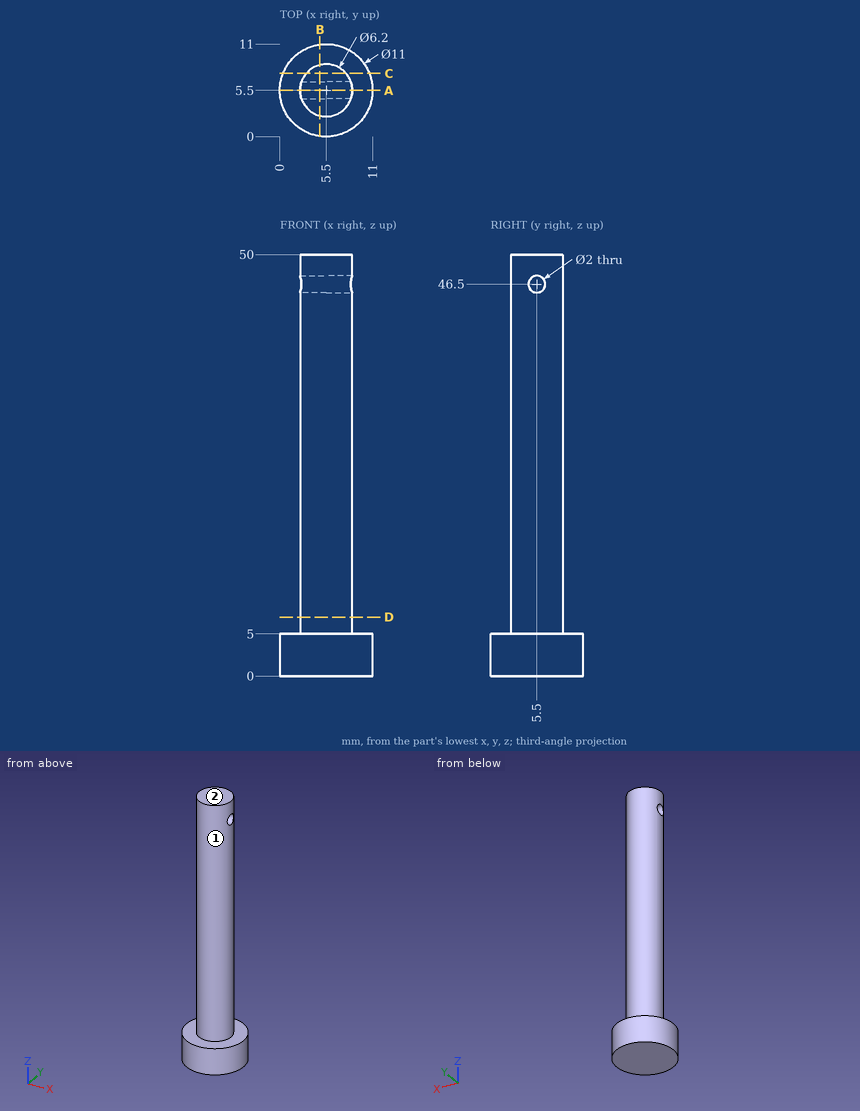
The figure shows three views and two pictorial views of one solid part (mm, origin at its lowest corner). Answer the questions. A direction names the side the tool comes from. Coordinates: 2 decimals unless noted, no trailing zeros. Order: outer loops, then holes, each group sorted by start corner. A loop starts at its lowest first (then second) coordinate and runs counter-clockwise, first axis right, second up.
Q1. A cutting plane is placed at D-D, the plane z = 7. Write down the section's boundary in (x, y), and give its area (3 significant figures).
Q2. Consider line 1 (Z direction, x = 4.35, y = 5.5); line 2 (Z direction, x = 1.5, y = 9); line 3 (Y direction, x = 5.5, z = 36). Determine where each line is inside the solid, lowest interval first.
Q3. Given P1, Ø2, axis at x = 6.5, z = 17.5, coming from the +Y side; P2, Ø3, axis at y = 5.5, z = 46.5, coming from the -X side; P3, Ø6, axis at x = 10, z = 32.5, coming from the +Y side; P4, Ø1.6, axis at y = 5.5, z = 46.5, coming from the +X side, each flat-ended and moving along its own axis, determine where each tip first touches the part or whether it passes through.
Q4. A cutting plane is placed at C-C, the plane y = 7.5. Write down the section's boundary in (x, z).
Q5. Which of the six approach directions +Z, -Z, +X, -X, +Y, -Y give full straight-line access (tool end or side, diameter ignored) to the marked faces 1 and 2?
Q6. A cutting plane is placed at B-B, the plane x = 4.75. Write down the section's boundary in (y, z), and give its area (3 significant figures).
Q7. A cutting plane is placed at A-A, the plane y = 5.5. Write down the section's boundary in (x, z), and give its area (3 significant figures).
Answers follow:
1. outline: circle Ø6.2 at (5.5, 5.5)
1. area: 30.2 mm2
2. line 1: z = 0 to 45.5, 47.5 to 50
2. line 2: z = 0 to 5
2. line 3: y = 2.4 to 8.6
3. P1: stops at y = 8.6
3. P2: stops at x = 2.4
3. P3: stops at y = 8.21
3. P4: passes through
4. outline: (0.38, 0) - (10.62, 0) - (10.62, 5) - (7.87, 5) - (7.87, 50) - (3.13, 50) - (3.13, 5) - (0.38, 5) - close
5. face 1: +Z
5. face 2: +Z, +X, -X, +Y, -Y
6. outline: (0.05, 0) - (10.95, 0) - (10.95, 5) - (8.51, 5) - (8.51, 50) - (2.49, 50) - (2.49, 5) - (0.05, 5) - close; hole circle Ø2 at (5.5, 46.5)
6. area: 322 mm2
7. outline: (0, 0) - (11, 0) - (11, 5) - (8.6, 5) - (8.6, 45.5) - (2.4, 45.5) - (2.4, 5) - (0, 5) - close; (2.4, 47.5) - (8.6, 47.5) - (8.6, 50) - (2.4, 50) - close
7. area: 322 mm2
